```python
from build123d import *

# Parameters (mm, degrees)
SKETCH_1_R          = 10
SKETCH_1_R_2        = 2.1
EXTRUDE_1_DEPTH     = 8
CUT_EXTRUDE_START   = -3
SKETCH_2_R          = 10
SKETCH_2_R_2        = 5
CUT_EXTRUDE_1_DEPTH = 2
FILLET_1_R          = 1
CUT_EXTRUDE_2_REACH = 18.248
SKETCH_3_R          = 1


with BuildPart() as part:
    # 草图1 → 凸台-拉伸1 (new body)
    with BuildSketch(Plane(origin=(0, 0, 0), x_dir=(1, 0, 0), z_dir=(0, 1, 0))):
        with Locations(Location((0, 0, 0), (0, 0, 270))):
            Circle(SKETCH_1_R)
        with Locations(Location((0, 0, 0), (0, 0, 270))):
            Circle(SKETCH_1_R_2, mode=Mode.SUBTRACT)
    extrude(amount=EXTRUDE_1_DEPTH)

    # 草图2 → 切除-拉伸1 (cut)
    with BuildSketch(Plane.XZ.offset(CUT_EXTRUDE_START)):
        with Locations(Location((0, 0, 0), (0, 0, 270))):
            Circle(SKETCH_2_R)
        with Locations(Location((0, 0, 0), (0, 0, 270))):
            Circle(SKETCH_2_R_2, mode=Mode.SUBTRACT)
    extrude(amount=-CUT_EXTRUDE_1_DEPTH, mode=Mode.SUBTRACT)

    # 圆角1
    fillet_1_edges = [part.edges().sort_by_distance(p)[0] for p in [
        (0, 5, 5),
        (0, 3, 5),
    ]]
    fillet(fillet_1_edges, radius=FILLET_1_R - 0.0001)  # a hair under: the kernel refuses the full size

    # 草图3 → 切除-拉伸2 (cut, up to next)
    with BuildSketch(Plane(origin=(0, 8, 0), x_dir=(1, 0, 0), z_dir=(0, 1, 0)), mode=Mode.PRIVATE) as cut_extrude_2_sk1:
        with Locations(Location((4.515189348, -5.349118166, 0), (0, 0, 270))):
            Circle(SKETCH_3_R)
    cut_extrude_2_tool1 = extrude(cut_extrude_2_sk1.sketch, amount=-CUT_EXTRUDE_2_REACH, mode=Mode.PRIVATE) & part.part
    add(cut_extrude_2_tool1.solids().sort_by_distance((4.515189, 8, 5.349118))[0], mode=Mode.SUBTRACT)


solid = part.part
```
The model under review builds one solid part; all positions refer to its coordinate system, in mm. A direction names the side the tool comes from. Round coordinates to 2 decimals unless told otherwise and drop trailing zeros. Loops run counter-clockwise (first coordinate to the right, second up) from the corner with the lowest first, then second, coordinate; pieces in that order, holes last. Notation, with made-up numbers: (36, 89) - (68, 89) arc R22 ccw to (68, 126) - close; hole circle Ø1 at (7.25, 84.25). An arc over 180 degrees is marked (long way). Write each question's results on one line, items separated by ' | '. Start each with the question number.
Q1. Tool access review of faces 1 (the flat face through (-7, 5, 0)), 2 (the cylindrical face through (4.13, 6.52, 6.27)), 3 (the cylindrical face through (0.631, 3.944, 2.003)): name each direction out of +Z, -Z, +X, -X, +Y, -Y from which nothing blocks a thin tool from reaching the whole face with its end or side.
Q2. Draft analysis for pull direction Y (two halves, no side actions). For faces 4 (the flat face through (-7, 3, 0)), 5 (the flat face through (2.4, 0, -0.1)), 6 (the flat face through (2.4, 8, -0.1)), state which applies: pulls with the +Y half, pulls with the -Y half, needs draft (parallel to the pull), parting line crosses it, or undercut.
Q3. Insertion check: P1, Ø1.5, axis at y = 7, z = -5.5, coming from the +X side; P2, Ø2, axis at x = 5.5, y = 3, coming from the -Z side; P3, Ø1.5, axis at y = 4, z = 2, coming from the -X side. Each pin has a flat end and moves straight along its axis. Give the tip position at first contact, or say it passes through.
Q4. Wall thickness on line 1 along Y through (x, z) = (7.75, -4); line 2 along X through (y, z) = (2.75, 0); line 3 along Z through (x, y) = (8, 6.75): over which ranges is each line inside the solid? List them lowest first. Write a range as [from, to].
Q5. Take a section at C-C on y = 0.5. Give the boundary of the cut face in (x, z).
Q6. Take a section at D-D on z = -9. Give the boundary of the cut face in (x, y), plus the area to 3 significant figures.
Data:
1) face 1: none | face 2: +Y | face 3: +Y, -Y
2) face 4: undercut | face 5: pulls with the -Y half | face 6: pulls with the +Y half
3) P1: stops at x = 8.8 | P2: stops at z = -8.93 | P3: stops at x = -5
4) line 1: y = [0, 3], [5, 8] | line 2: x = [-10, -2.1], [2.1, 10] | line 3: z = [-6, 6]
5) outline: circle Ø20 at (0, 0); hole circle Ø4.2 at (0, 0)
6) outline: (-4.36, 0) - (4.36, 0) - (4.36, 3) - (-4.36, 3) - close; (-4.36, 5) - (4.36, 5) - (4.36, 8) - (-4.36, 8) - close | area: 52.3 mm²
